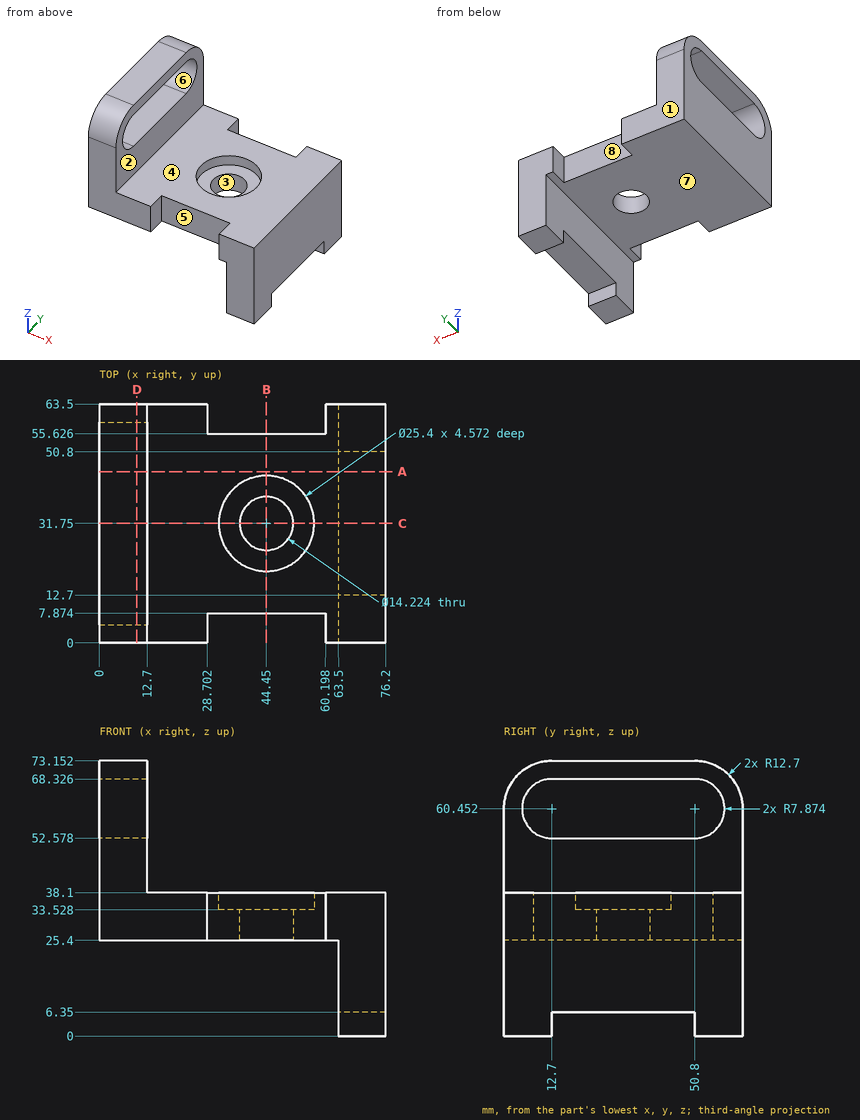
Geometry: see drawing. Coordinates: mm, zero at the bounding-box minimum. A direction names the side the tool comes from. Give positions to 0.01 mm unless a question says otherwise; leave off trailing zeros. Loops run counter-clockwise (first coordinate to the right, second up) from the corner with the lowest first, then second, coordinate; pieces in that order, holes last. Notation, with made-up numbers: (63, 3.25) - (115, 3.25) arc R18 ccw to (115, 33.25) - close; hole circle Ø5 at (42.5, -10). An arc over 180 degrees is marked (long way). One line per question, with ' | ' between items. Start each with the question number.
(1) Section query B-B on x = 44.45. Return loops of the section in (y, z).
(2) Contact query for flat-ended pins moving along their axis: pin 1 (11.5 mm diameter, centred on x = 44.45, y = 31.75, fed in from -Z); pin 2 (8 mm diameter, centred on x = 28.5, y = 39, fed in from +Z); pin 3 (14 mm diameter, centred on x = 51.5, z = 31, fed in from +Y); pin 4 (1.5 mm diameter, centred on y = 39.5, z = 14, fed in from -X). Output: stop coordinate, or through.
(3) Reachability of the marked faces 4, 5, 6, 7 and 8 from +Z, -Z, +X, -X, +Y, -Y: full face, straight path, thin tool, end or side. Return the list, or none.
(4) Pull-direction query (X, two-part tool) for the marked faces 1, 2 and 3; classes: released by +X, released by -X, zero draft, split by the parting line, or undercut.
(5) Section query A-A on y = 45.5. Return loops of the section in (x, z).
(6) Section query D-D on x = 10. Return loops of the section in (y, z), then the cut area to 3 significant figures.
(7) Ray query, line 1 (Y direction, x = 44, z = 35); line 2 (Y direction, x = 44, z = 28); line 3 (X direction, y = 7, z = 30). Return the intervals inside material, ascending. Write a range as from..to.
(8) Section query C-C on y = 31.75. Return loops of the section in (x, z).
The answers:
1) outline: (7.87, 25.4) - (24.64, 25.4) - (24.64, 33.53) - (19.05, 33.53) - (19.05, 38.1) - (7.87, 38.1) - close; (38.86, 25.4) - (55.63, 25.4) - (55.63, 38.1) - (44.45, 38.1) - (44.45, 33.53) - (38.86, 33.53) - close
2) pin 1: through | pin 2: z = 38.1 | pin 3: y = 55.63 | pin 4: x = 63.5
3) face 4: +Z, +X, +Y, -Y | face 5: +Z, -Z, -Y | face 6: +X, -X | face 7: -Z, -X, +Y, -Y | face 8: +Z, -Z, +Y
4) face 1: zero draft | face 2: released by +X | face 3: undercut
5) outline: (0, 25.4) - (63.5, 25.4) - (63.5, 6.35) - (76.2, 6.35) - (76.2, 38.1) - (12.7, 38.1) - (12.7, 52.58) - (0, 52.58) - close; (0, 68.33) - (12.7, 68.33) - (12.7, 73.15) - (0, 73.15) - close
6) outline: (0, 25.4) - (63.5, 25.4) - (63.5, 60.45) arc R12.7 ccw to (50.8, 73.15) - (12.7, 73.15) arc R12.7 ccw to (0, 60.45) - close; hole (12.7, 52.58) - (50.8, 52.58) arc R7.87 ccw to (50.8, 68.33) - (12.7, 68.33) arc R7.87 ccw to start | area: 2,170 mm2
7) line 1: 7.87..19.06, 44.44..55.63 | line 2: 7.87..24.65, 38.85..55.63 | line 3: 0..28.7, 60.2..76.2
8) outline: (0, 25.4) - (37.34, 25.4) - (37.34, 33.53) - (31.75, 33.53) - (31.75, 38.1) - (12.7, 38.1) - (12.7, 52.58) - (0, 52.58) - close; (0, 68.33) - (12.7, 68.33) - (12.7, 73.15) - (0, 73.15) - close; (51.56, 25.4) - (63.5, 25.4) - (63.5, 6.35) - (76.2, 6.35) - (76.2, 38.1) - (57.15, 38.1) - (57.15, 33.53) - (51.56, 33.53) - close
